```python
from build123d import *

# Parameters (mm, degrees)
SKETCH1_R           = 10
BOSS_EXTRUDE1_DEPTH = 30
BOSS_EXTRUDE2_DEPTH = 100


with BuildPart() as part:
    # Sketch1 → Boss-Extrude1 (new body, symmetric)
    with BuildSketch(Plane.XY):
        Circle(SKETCH1_R)
    extrude(amount=BOSS_EXTRUDE1_DEPTH, both=True)

    # Sketch2 → Boss-Extrude2 (add)
    with BuildSketch(Plane.XY.offset(30)):
        with BuildLine():
            ThreePointArc((2.305037087, 19.866726052), (0, 20), (-2.305037087, 19.866726052))
            Line((-2.305037087, 19.866726052), (-4, 9.16515139))
            ThreePointArc((-4, 9.16515139), (-5.877852523, 8.090169944), (-7.480508975, 6.636413601))
            Line((-7.480508975, 6.636413601), (-18.182083637, 8.331376514))
            ThreePointArc((-18.182083637, 8.331376514), (-19.021130326, 6.180339887), (-19.606674902, 3.946935431))
            Line((-19.606674902, 3.946935431), (-9.95264493, -0.97203853))
            ThreePointArc((-9.95264493, -0.97203853), (-9.510565163, -3.090169944), (-8.6232088, -5.063622221))
            Line((-8.6232088, -5.063622221), (-13.54218276, -14.717652193))
            ThreePointArc((-13.54218276, -14.717652193), (-11.755705046, -16.180339887), (-9.812554409, -17.427385804))
            Line((-9.812554409, -17.427385804), (-2.151072845, -9.76590424))
            ThreePointArc((-2.151072845, -9.76590424), (0, -10), (2.151072845, -9.76590424))
            Line((2.151072845, -9.76590424), (9.812554409, -17.427385804))
            ThreePointArc((9.812554409, -17.427385804), (11.755705046, -16.180339887), (13.54218276, -14.717652193))
            Line((13.54218276, -14.717652193), (8.6232088, -5.063622221))
            ThreePointArc((8.6232088, -5.063622221), (9.510565163, -3.090169944), (9.95264493, -0.97203853))
            Line((9.95264493, -0.97203853), (19.606674902, 3.946935431))
            ThreePointArc((19.606674902, 3.946935431), (19.021130326, 6.180339887), (18.182083637, 8.331376514))
            Line((18.182083637, 8.331376514), (7.480508975, 6.636413601))
            ThreePointArc((7.480508975, 6.636413601), (5.877852523, 8.090169944), (4, 9.16515139))
            Line((4, 9.16515139), (2.305037087, 19.866726052))
        make_face()
    extrude(amount=BOSS_EXTRUDE2_DEPTH)


solid = part.part
```
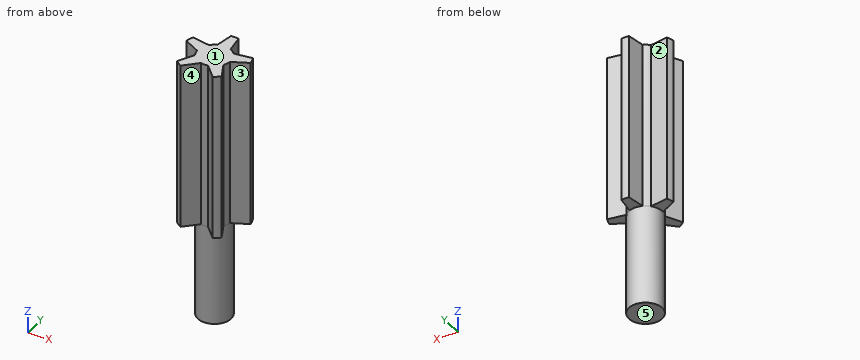
Read the model definition and answer for the solid it produces. Units are mm, in the model's axes. Face numbers are marked on the shaded views. A direction names the side the tool comes from. Give positions to 0.01 mm unless a question says otherwise; leave off trailing zeros. Write each loop counter-clockwise with the first axis right and the second up, starting at its lowest first coordinate (ties: lowest second). Pieces come first, ordered by that corner, then holes. Notation, with made-up numbers: (-25, 22) -> (32, 22) arc R29 ccw to (32, 45) -> close; hole circle Ø10 at (-23.5, 66.25). An arc over 180 degrees is marked (long way). Answer as a JSON object with one key per item and string values.
1) Section C-C on x = 0 is taken. Write down the section's boundary in (y, z), then the cut area to 3 significant figures.
Findings below:
{"outline": "(-10, -30) -> (10, -30) -> (10, 30) -> (20, 30) -> (20, 130) -> (-10, 130) -> close", "area": "4,200 mm^2"}
2) For a pull along X with two mould halves and no side action, classify the marked faces 3, 4 and 5 as pulls with the +X half, pulls with the -X half, needs draft (parallel to the pull), parting line crosses it, or undercut.
Findings below:
{"face 3": "pulls with the +X half", "face 4": "undercut", "face 5": "needs draft"}
3) Straight lines are drawn through the part: probe 1 along Y at (x, z) = (-0.5, 36); probe 2 along Z at (x, y) = (12, -15); probe 3 along X at (y, z) = (-14, 34). For each, find the intervals that lie inside material, in ascending order. Write a range as from..to.
Findings below:
{"probe 1": "y = -9.99..19.99", "probe 2": "z = 30..130", "probe 3": "x = -13.18..-6.39, 6.39..13.18"}
4) Section B-B on z = 33.5 is taken. Write down the section's boundary in (x, y), then the cut area to 3 significant figures.
Findings below:
{"outline": "(-19.61, 3.95) -> (-9.95, -0.97) arc R10 ccw to (-8.62, -5.06) -> (-13.54, -14.72) arc R20 ccw to (-9.81, -17.43) -> (-2.15, -9.77) arc R10 ccw to (2.15, -9.77) -> (9.81, -17.43) arc R20 ccw to (13.54, -14.72) -> (8.62, -5.06) arc R10 ccw to (9.95, -0.97) -> (19.61, 3.95) arc R20 ccw to (18.18, 8.33) -> (7.48, 6.64) arc R10 ccw to (4, 9.17) -> (2.31, 19.87) arc R20 ccw to (-2.31, 19.87) -> (-4, 9.17) arc R10 ccw to (-7.48, 6.64) -> (-18.18, 8.33) arc R20 ccw to start", "area": "631 mm^2"}
5) A tool of negligible diameter and unlimited length cuts with its end or side. For the marked faces 1 and 2, from which of +Z, -Z, +X, -X, +Y, -Y can it reach the whole face along a straight path? Write none if from no direction.
Findings below:
{"face 1": "+Z, +X, -X, +Y, -Y", "face 2": "+Z, -Z, +Y"}
6) Section A-A on x = -11.5 is taken. Write down the section's boundary in (y, z), then the cut area to 3 significant figures.
Findings below:
{"outline": "(-16.36, 30) -> (-10.71, 30) -> (-10.71, 130) -> (-16.36, 130) -> close; (-0.18, 30) -> (7.27, 30) -> (7.27, 130) -> (-0.18, 130) -> close", "area": "1,310 mm^2"}
7) Flat-ended cylindrical pins translate along their axes: pin 1 Ø10 at (x, y) = (14, 5.5) entering from -Z; pin 2 Ø6 at (x, z) = (-11, 45.5) entering from -Y; pin 3 Ø4 at (y, z) = (11.5, 68) entering from -X; pin 4 Ø8 at (y, z) = (-5.5, 56) entering from -X. Find the tip coordinate at first contact, or state that the pin passes through.
Findings below:
{"pin 1": "stops at z = 30", "pin 2": "stops at y = -17.43", "pin 3": "stops at x = -3.95", "pin 4": "stops at x = -10.88"}
8) Section D-D on y = -3.5 is taken. Write down the section's boundary in (x, z), then the cut area to 3 significant figures.
Findings below:
{"outline": "(-9.37, -30) -> (9.37, -30) -> (9.37, 130) -> (-9.37, 130) -> close", "area": "3,000 mm^2"}
